Can you work these out from the model? Positions are in its coordinate system, mm. Give positions to 0.01 mm unless a question says otherwise; leave off trailing zeros. Loops run counter-clockwise (first coordinate to the right, second up) from the corner with the lowest first, then second, coordinate; pieces in that order, holes last. Notation, with made-up numbers: (15, 47) - (38, 47) arc R24 cw to (38, 66) - close; hole circle Ø7 at (24, 38). An arc over 180 degrees is marked (long way). Answer as a JSON object with one key per item and string values.
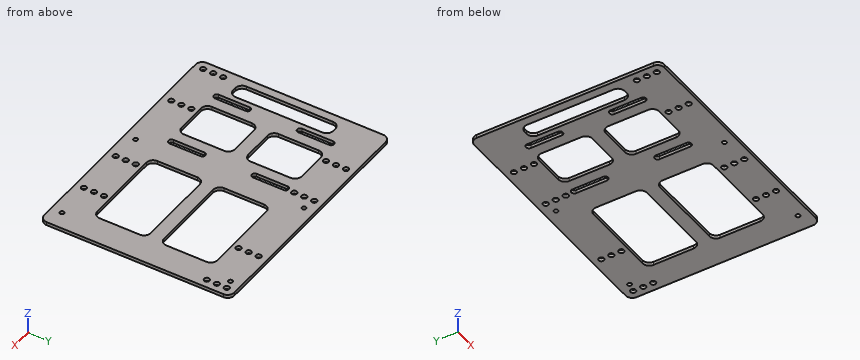
```python
from build123d import *

# Parameters (mm, degrees)
BOSS_EXTRUDE1_DEPTH     = 2
CUT_EXTRUDE6_DEPTH      = 95.223139409
CUT_EXTRUDE6_DEPTH_BACK = 95.223139409
SKETCH2_R               = 1.6
SKETCH2_R_2             = 1.25


with BuildPart() as part:
    # Sketch1 → Boss-Extrude1 (new body)
    with BuildSketch(Plane(origin=(0, 0, 0), x_dir=(0, 1, 0), z_dir=(0, 0, 1))):
        with BuildLine():
            Line((-53, -75), (53, -75))
            ThreePointArc((53, -75), (55.828427125, -73.828427125), (57, -71))
            Line((57, -71), (57, 71))
            ThreePointArc((57, 71), (55.828427125, 73.828427125), (53, 75))
            Line((53, 75), (-53, 75))
            ThreePointArc((-53, 75), (-55.828427125, 73.828427125), (-57, 71))
            Line((-57, 71), (-57, -71))
            ThreePointArc((-57, -71), (-55.828427125, -73.828427125), (-53, -75))
        make_face()
    extrude(amount=BOSS_EXTRUDE1_DEPTH)

    # Sketch2 → Cut-Extrude6 (cut, two sides: drawn at the far end of the back side and taken through both)
    with BuildSketch(Plane(origin=(0, 0, 0), x_dir=(0, 1, 0), z_dir=(0, 0, 1)).offset(-CUT_EXTRUDE6_DEPTH_BACK)):
        with Locations(Location((-51.8, 40.1, 0), (0, 0, 270))):
            Circle(SKETCH2_R)
        with Locations(Location((-51.8, 69.9, 0), (0, 0, 270))):
            Circle(SKETCH2_R)
        with Locations(Location((-45.8, 40.1, 0), (0, 0, 270))):
            Circle(SKETCH2_R)
        with Locations(Location((-45.8, 69.9, 0), (0, 0, 270))):
            Circle(SKETCH2_R)
        with Locations(Location((-39.8, 40.1, 0), (0, 0, 270))):
            Circle(SKETCH2_R)
        with Locations(Location((-39.8, 69.9, 0), (0, 0, 270))):
            Circle(SKETCH2_R)
        with Locations(Location((-51.8, -41.9, 0), (0, 0, 270))):
            Circle(SKETCH2_R)
        with Locations(Location((-51.8, -12.1, 0), (0, 0, 270))):
            Circle(SKETCH2_R)
        with Locations(Location((-45.8, -41.9, 0), (0, 0, 270))):
            Circle(SKETCH2_R)
        with Locations(Location((-45.8, -12.1, 0), (0, 0, 270))):
            Circle(SKETCH2_R)
        with Locations(Location((-39.8, -41.9, 0), (0, 0, 270))):
            Circle(SKETCH2_R)
        with Locations(Location((-39.8, -12.1, 0), (0, 0, 270))):
            Circle(SKETCH2_R)
        with Locations(Location((51.8, 12.1, 0), (0, 0, 270))):
            Circle(SKETCH2_R)
        with Locations(Location((51.8, 41.9, 0), (0, 0, 270))):
            Circle(SKETCH2_R)
        with Locations(Location((45.8, 12.1, 0), (0, 0, 270))):
            Circle(SKETCH2_R)
        with Locations(Location((45.8, 41.9, 0), (0, 0, 270))):
            Circle(SKETCH2_R)
        with Locations(Location((39.8, 12.1, 0), (0, 0, 270))):
            Circle(SKETCH2_R)
        with Locations(Location((39.8, 41.9, 0), (0, 0, 270))):
            Circle(SKETCH2_R)
        with Locations(Location((51.8, -69.9, 0), (0, 0, 270))):
            Circle(SKETCH2_R)
        with Locations(Location((51.8, -40.1, 0), (0, 0, 270))):
            Circle(SKETCH2_R)
        with Locations(Location((45.8, -69.9, 0), (0, 0, 270))):
            Circle(SKETCH2_R)
        with Locations(Location((45.8, -40.1, 0), (0, 0, 270))):
            Circle(SKETCH2_R)
        with Locations(Location((39.8, -69.9, 0), (0, 0, 270))):
            Circle(SKETCH2_R)
        with Locations(Location((39.8, -40.1, 0), (0, 0, 270))):
            Circle(SKETCH2_R)
        with Locations(Location((-50.5, -64.5, 0), (0, 0, 270))):
            Circle(SKETCH2_R_2)
        with Locations(Location((-50.5, 4.5, 0), (0, 0, 270))):
            Circle(SKETCH2_R_2)
        with Locations(Location((50.5, -64.5, 0), (0, 0, 270))):
            Circle(SKETCH2_R_2)
        with Locations(Location((50.5, 4.5, 0), (0, 0, 270))):
            Circle(SKETCH2_R_2)
        with BuildLine():
            Line((-34.3, 11), (-15.7, 11))
            ThreePointArc((-15.7, 11), (-14.497918472, 11.497918472), (-14, 12.7))
            Line((-14, 12.7), (-14, 12.8))
            ThreePointArc((-14, 12.8), (-14.497918472, 14.002081528), (-15.7, 14.5))
            Line((-15.7, 14.5), (-34.3, 14.5))
            ThreePointArc((-34.3, 14.5), (-35.502081528, 14.002081528), (-36, 12.8))
            Line((-36, 12.8), (-36, 12.7))
            ThreePointArc((-36, 12.7), (-35.502081528, 11.497918472), (-34.3, 11))
        make_face()
        with BuildLine():
            Line((-34.3, 53.5), (-15.7, 53.5))
            ThreePointArc((-15.7, 53.5), (-14.497918472, 53.997918472), (-14, 55.2))
            Line((-14, 55.2), (-14, 55.3))
            ThreePointArc((-14, 55.3), (-14.497918472, 56.502081528), (-15.7, 57))
            Line((-15.7, 57), (-34.3, 57))
            ThreePointArc((-34.3, 57), (-35.502081528, 56.502081528), (-36, 55.3))
            Line((-36, 55.3), (-36, 55.2))
            ThreePointArc((-36, 55.2), (-35.502081528, 53.997918472), (-34.3, 53.5))
        make_face()
        with BuildLine():
            Line((15.7, 11), (34.3, 11))
            ThreePointArc((34.3, 11), (35.502081528, 11.497918472), (36, 12.7))
            Line((36, 12.7), (36, 12.8))
            ThreePointArc((36, 12.8), (35.502081528, 14.002081528), (34.3, 14.5))
            Line((34.3, 14.5), (15.7, 14.5))
            ThreePointArc((15.7, 14.5), (14.497918472, 14.002081528), (14, 12.8))
            Line((14, 12.8), (14, 12.7))
            ThreePointArc((14, 12.7), (14.497918472, 11.497918472), (15.7, 11))
        make_face()
        with BuildLine():
            Line((15.7, 53.5), (34.3, 53.5))
            ThreePointArc((34.3, 53.5), (35.502081528, 53.997918472), (36, 55.2))
            Line((36, 55.2), (36, 55.3))
            ThreePointArc((36, 55.3), (35.502081528, 56.502081528), (34.3, 57))
            Line((34.3, 57), (15.7, 57))
            ThreePointArc((15.7, 57), (14.497918472, 56.502081528), (14, 55.3))
            Line((14, 55.3), (14, 55.2))
            ThreePointArc((14, 55.2), (14.497918472, 53.997918472), (15.7, 53.5))
        make_face()
        with BuildLine():
            Line((-32, -58), (-8, -58))
            ThreePointArc((-8, -58), (-5.171572875, -56.828427125), (-4, -54))
            Line((-4, -54), (-4, -8))
            ThreePointArc((-4, -8), (-5.171572875, -5.171572875), (-8, -4))
            Line((-8, -4), (-32, -4))
            ThreePointArc((-32, -4), (-34.828427125, -5.171572875), (-36, -8))
            Line((-36, -8), (-36, -54))
            ThreePointArc((-36, -54), (-34.828427125, -56.828427125), (-32, -58))
        make_face()
        with BuildLine():
            Line((-32, 21), (-8, 21))
            ThreePointArc((-8, 21), (-5.171572875, 22.171572875), (-4, 25))
            Line((-4, 25), (-4, 43))
            ThreePointArc((-4, 43), (-5.171572875, 45.828427125), (-8, 47))
            Line((-8, 47), (-32, 47))
            ThreePointArc((-32, 47), (-34.828427125, 45.828427125), (-36, 43))
            Line((-36, 43), (-36, 25))
            ThreePointArc((-36, 25), (-34.828427125, 22.171572875), (-32, 21))
        make_face()
        with BuildLine():
            Line((8, -58), (32, -58))
            ThreePointArc((32, -58), (34.828427125, -56.828427125), (36, -54))
            Line((36, -54), (36, -8))
            ThreePointArc((36, -8), (34.828427125, -5.171572875), (32, -4))
            Line((32, -4), (8, -4))
            ThreePointArc((8, -4), (5.171572875, -5.171572875), (4, -8))
            Line((4, -8), (4, -54))
            ThreePointArc((4, -54), (5.171572875, -56.828427125), (8, -58))
        make_face()
        with BuildLine():
            Line((8, 21), (32, 21))
            ThreePointArc((32, 21), (34.828427125, 22.171572875), (36, 25))
            Line((36, 25), (36, 43))
            ThreePointArc((36, 43), (34.828427125, 45.828427125), (32, 47))
            Line((32, 47), (8, 47))
            ThreePointArc((8, 47), (5.171572875, 45.828427125), (4, 43))
            Line((4, 43), (4, 25))
            ThreePointArc((4, 25), (5.171572875, 22.171572875), (8, 21))
        make_face()
        with BuildLine():
            Line((-26, 60), (26, 60))
            ThreePointArc((26, 60), (28.828427125, 61.171572875), (30, 64))
            Line((30, 64), (30, 66))
            ThreePointArc((30, 66), (28.828427125, 68.828427125), (26, 70))
            Line((26, 70), (-26, 70))
            ThreePointArc((-26, 70), (-28.828427125, 68.828427125), (-30, 66))
            Line((-30, 66), (-30, 64))
            ThreePointArc((-30, 64), (-28.828427125, 61.171572875), (-26, 60))
        make_face()
    extrude(amount=CUT_EXTRUDE6_DEPTH + CUT_EXTRUDE6_DEPTH_BACK, mode=Mode.SUBTRACT)


solid = part.part
```
1) Imagine slicing it at A-A on y = -45.8. Write out the boundary of the cut face in (x, z), and give its area (3 significant figures).
Check sheet entries:
{"outline": "(-75, 0) - (-71.5, 0) - (-71.5, 2) - (-75, 2) - close; (-68.3, 0) - (-41.7, 0) - (-41.7, 2) - (-68.3, 2) - close; (-38.5, 0) - (10.5, 0) - (10.5, 2) - (-38.5, 2) - close; (13.7, 0) - (40.3, 0) - (40.3, 2) - (13.7, 2) - close; (43.5, 0) - (75, 0) - (75, 2) - (43.5, 2) - close", "area": "274 mm2"}
2) I need wall thicknesses on L1, parallel to Y at x = 41.9, z = 1.15; L2, parallel to X at y = -9, z = 1; L3, parallel to X at y = 15.5, z = 0.8. Which ranges of each line are inside material? Lowest first, please.
Check sheet entries:
{"L1": "-57 to -53.4, -50.2 to -47.4, -44.2 to -41.4, -38.2 to -36, -4 to 4, 36 to 57", "L2": "-75 to -70, -60 to -47, -21 to 4, 58 to 75", "L3": "-75 to -70, -60 to -56.99, -53.51 to -47, -21 to -14.49, -11.01 to 4, 58 to 75"}
3) Imagine slicing it at D-D on z = 0.35. Give the number of separate pieces and of enclosed holes in the cut face, and give its area (3 significant figures).
Check sheet entries:
{"separate pieces": "1", "enclosed holes": "37", "area": "10,900 mm2"}
4) Imagine slicing it at C-C on y = -6. Write out the boundary of the cut face in (x, z).
Check sheet entries:
{"outline": "(-75, 0) - (-70, 0) - (-70, 2) - (-75, 2) - close; (-60, 0) - (-46.46, 0) - (-46.46, 2) - (-60, 2) - close; (-21.54, 0) - (4.54, 0) - (4.54, 2) - (-21.54, 2) - close; (57.46, 0) - (75, 0) - (75, 2) - (57.46, 2) - close"}
5) I'm going to push a flat-ended pin straight in: P1, Ø3.5, axis at x = -69.9, y = -45.8, coming from the -Z side. Where does the tip first touch, or does it pass through?
Check sheet entries:
{"P1": "z = 0"}
6) Imagine slicing it at B-B on x = 21. Write out the boundary of the cut face in (y, z), and give its area (3 significant figures).
Check sheet entries:
{"outline": "(-57, 0) - (-36, 0) - (-36, 2) - (-57, 2) - close; (-4, 0) - (4, 0) - (4, 2) - (-4, 2) - close; (36, 0) - (57, 0) - (57, 2) - (36, 2) - close", "area": "100 mm2"}
